Part print with two shaded views. Sizes in mm from the minimum x, y, z corner. Give positions to 0.01 mm unless a question says otherwise; leave off trailing zeros. Write each loop counter-clockwise with the first axis right and the second up, starting at its lowest first coordinate (ties: lowest second). Pieces come first, ordered by that corner, then holes. Notation, with made-up numbers: (-27.5, 36.25) - (18.5, 36.25) arc R21 ccw to (18.5, 42.25) - close; hole circle Ø2 at (71, 46.5). An arc over 180 degrees is marked (long way). One line per item, written item: value. Start each with the question number.
(1) Cut at C-C, the plane y = 1.5. List the corners of the cut face in (x, z) (1 decimal).
(2) Drop a flat-ended pin along its axis: P1, Ø6.5, axis at x = 43, y = 7.5, coming from the +Z side. Give the stop position or say it passes through.
(3) Cut at D-D, the plane x = 57. List the corners of the cut face in (y, z).
(4) Cut at B-B, the plane y = 6.35. List the corners of the cut face in (x, z) (1 decimal).
(5) Cut at A-A, the plane z = 6.25. List the corners of the cut face in (x, y).
(6) Probe L1, parallel to Z at x = 30.5, y = 1.5; L2, parallel to X at y = 8, z = 7.75; L3, parallel to Z at x = 4, y = 7.5 (1 decimal). List the from-to ranges inside material, lowest first.
(7) Mould opens along Y. For the marked faces 1, 2, 3 and 4 say: pulls with the +Y half, pulls with the -Y half, needs draft (parallel to the pull), parting line crosses it, or undercut.
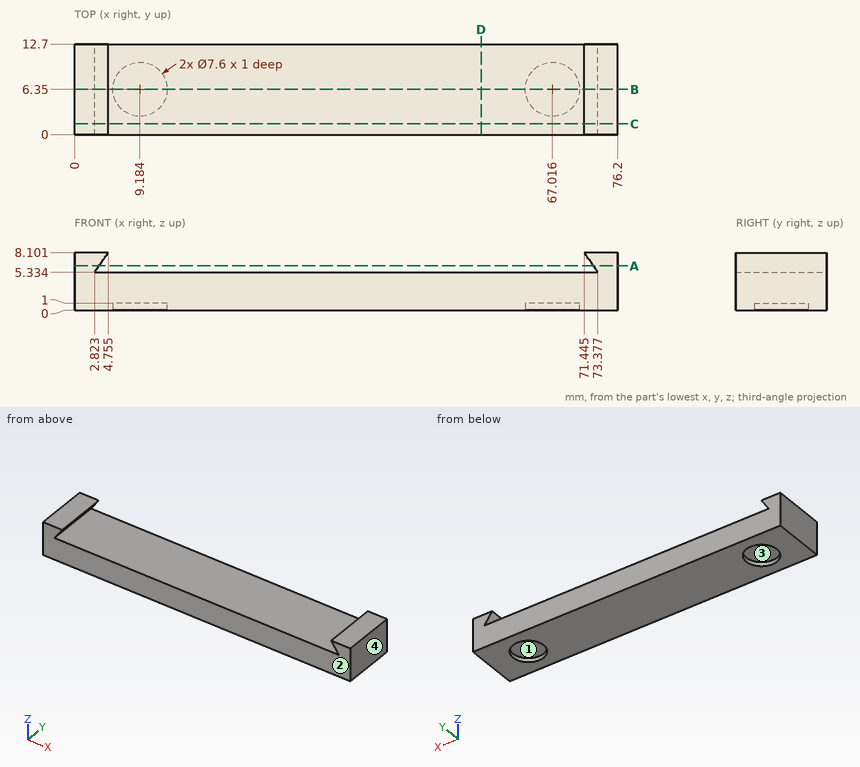
Answers follow:
1. outline: (0, 0) - (76.2, 0) - (76.2, 8.1) - (71.4, 8.1) - (73.4, 5.3) - (2.8, 5.3) - (4.8, 8.1) - (0, 8.1) - close
2. P1: stops at z = 5.33
3. outline: (0, 0) - (12.7, 0) - (12.7, 5.33) - (0, 5.33) - close
4. outline: (0, 0) - (5.4, 0) - (5.4, 1) - (13, 1) - (13, 0) - (63.2, 0) - (63.2, 1) - (70.8, 1) - (70.8, 0) - (76.2, 0) - (76.2, 8.1) - (71.4, 8.1) - (73.4, 5.3) - (2.8, 5.3) - (4.8, 8.1) - (0, 8.1) - close
5. outline: (0, 0) - (3.46, 0) - (3.46, 12.7) - (0, 12.7) - close; (72.74, 0) - (76.2, 0) - (76.2, 12.7) - (72.74, 12.7) - close
6. L1: z = 0 to 5.33
6. L2: x = 0 to 4.51, 71.69 to 76.2
6. L3: z = 0 to 5.3, 7 to 8.1
7. face 1: undercut
7. face 2: pulls with the -Y half
7. face 3: undercut
7. face 4: needs draft
